```python
from build123d import *

# Parameters (mm, degrees)
SKETCH1_R           = 37.5
BOSS_EXTRUDE1_DEPTH = 2
SKETCH2_R           = 3
BOSS_EXTRUDE2_DEPTH = 5
SKETCH3_R           = 2.5
CUT_EXTRUDE1_DEPTH  = 3
BOSS_EXTRUDE3_DEPTH = 80
SKETCH5_R           = 37.5
SKETCH5_R_2         = 2.75
BOSS_EXTRUDE4_DEPTH = 2


with BuildPart() as part:
    # Sketch1 → Boss-Extrude1 (new body)
    with BuildSketch(Plane(origin=(0, 0, 0), x_dir=(1, 0, 0), z_dir=(0, 1, 0))):
        with Locations(Location((0, 0, 0), (0, 0, 270))):
            Circle(SKETCH1_R)
    extrude(amount=BOSS_EXTRUDE1_DEPTH)

    # Sketch2 → Boss-Extrude2 (add)
    with BuildSketch(Plane(origin=(0, 2, 0), x_dir=(1, 0, 0), z_dir=(0, 1, 0))):
        with Locations(Location((0, 0, 0), (0, 0, 270))):
            Circle(SKETCH2_R)
    extrude(amount=BOSS_EXTRUDE2_DEPTH)

    # Sketch3 → Cut-Extrude1 (cut)
    with BuildSketch(Plane(origin=(0, 7, 0), x_dir=(1, 0, 0), z_dir=(0, 1, 0))):
        with Locations(Location((0, 0, 0), (0, 0, 270))):
            Circle(SKETCH3_R)
    extrude(amount=-CUT_EXTRUDE1_DEPTH, mode=Mode.SUBTRACT)

    # Sketch4 → Boss-Extrude3 (add)
    with BuildSketch(Plane(origin=(0, 2, 0), x_dir=(1, 0, 0), z_dir=(0, 1, 0))):
        with BuildLine():
            Line((-37.5, 0), (-36.5, 0))
            ThreePointArc((-36.5, 0), (0, 36.5), (36.5, 0))
            Line((36.5, 0), (37.5, 0))
            ThreePointArc((37.5, 0), (0, 37.5), (-37.5, 0))
        make_face()
    extrude(amount=BOSS_EXTRUDE3_DEPTH)

    # Sketch5 → Boss-Extrude4 (add)
    with BuildSketch(Plane(origin=(0, 82, 0), x_dir=(1, 0, 0), z_dir=(0, 1, 0))):
        with Locations(Location((0, 0, 0), (0, 0, 270))):
            Circle(SKETCH5_R)
        with Locations(Location((0, 0, 0), (0, 0, 270))):
            Circle(SKETCH5_R_2, mode=Mode.SUBTRACT)
    extrude(amount=BOSS_EXTRUDE4_DEPTH)


solid = part.part
```
CAD build for the part. Positions are in the model's coordinates, mm. A direction names the side the tool comes from. Round coordinates to 2 decimals unless told otherwise and drop trailing zeros. Order: outer loops, then holes, each group sorted by start corner. A loop starts at its lowest first (then second) coordinate and runs counter-clockwise, first axis right, second up. Notation, with made-up numbers: (45.5, 74) -> (58.5, 74) arc R13 ccw to (58.5, 83) -> close; hole circle Ø8 at (83.25, 33.5). An arc over 180 degrees is marked (long way). One line per question, with ' | ' between items.
Q1. Slice it at C-C (z = -13.5). Write the cut outline in (x, y), then the cut area to 3 significant figures.
Completed:
outline: (-34.99, 0) -> (34.99, 0) -> (34.99, 84) -> (-34.99, 84) -> close; hole (-33.91, 2) -> (33.91, 2) -> (33.91, 82) -> (-33.91, 82) -> close | area: 452 mm^2
Q2. Slice it at D-D (x = 15). Write the cut outline in (y, z).
Completed:
outline: (0, -34.37) -> (84, -34.37) -> (84, 34.37) -> (82, 34.37) -> (82, -33.28) -> (2, -33.28) -> (2, 34.37) -> (0, 34.37) -> close
Q3. Two-plate mould, pull along X, no slides. Class faces 4 (the cylindrical face through (1.649, 41.412, -37.464)), 5 (the flat face through (1, 0, -1)), 6 (the flat face through (2, 7, -2)): released by +X, released by -X, zero draft, split by the parting line, or undercut.
Completed:
face 4: split by the parting line | face 5: zero draft | face 6: undercut
Q4. Slice it at B-B (z = 8.5). Write the cut outline in (x, y).
Completed:
outline: (-36.52, 0) -> (36.52, 0) -> (36.52, 2) -> (-36.52, 2) -> close; (-36.52, 82) -> (36.52, 82) -> (36.52, 84) -> (-36.52, 84) -> close
Q5. Which spindle directions (+Z, -Z, +X, -X, +Y, -Y) get a long thin tool onto all of the face, cutting with end or side? Do faces 1 (the cylindrical face through (0.9, 4.46, 2.86)), 2 (the flat face through (0, 4, 0)), 3 (the flat face through (1, 82, 8)). Say none if no direction does.
Completed:
face 1: none | face 2: +Y | face 3: +Z
Q6. Drop flat-ended pins along their axis: pin 1 (8 mm diameter, centred on y = 38, z = -25.5, fed in from -X); pin 2 (6 mm diameter, centred on x = 21.5, y = 68, fed in from +Z); pin 3 (3 mm diameter, centred on x = 0, z = 0, fed in from +Y). Give the stop position or say it passes through.
Completed:
pin 1: stops at x = -30.72 | pin 2: stops at z = -27.06 | pin 3: stops at y = 4
Q7. Probe probe 1 along Y at (x, z) = (-9, -17.5); probe 2 along X at (y, z) = (83.6, 0); probe 3 along Y at (x, z) = (-2, 2). List the from-to ranges inside material, lowest first.
Completed:
probe 1: y = 0 to 2, 82 to 84 | probe 2: x = -37.5 to -2.75, 2.75 to 37.5 | probe 3: y = 0 to 7, 82 to 84
Q8. Slice it at A-A (x = 0). Write the cut outline in (y, z).
Completed:
outline: (0, -37.5) -> (84, -37.5) -> (84, -2.75) -> (82, -2.75) -> (82, -36.5) -> (2, -36.5) -> (2, -3) -> (7, -3) -> (7, -2.5) -> (4, -2.5) -> (4, 2.5) -> (7, 2.5) -> (7, 3) -> (2, 3) -> (2, 37.5) -> (0, 37.5) -> close; (82, 2.75) -> (84, 2.75) -> (84, 37.5) -> (82, 37.5) -> close
